The figure shows three views and two pictorial views of one solid part (mm, origin at its lowest corner). Answer the questions. Round coordinates to 2 decimals unless told otherwise and drop trailing zeros. Order: outer loops, then holes, each group sorted by start corner. A loop starts at its lowest first (then second) coordinate and runs counter-clockwise, first axis right, second up. Notation, with made-up numbers: (-14.5, 86.25) - (32.5, 86.25) arc R24 cw to (32.5, 104.25) - close; hole circle Ø6 at (75.5, 53). An arc over 180 degrees is marked (long way). One line per item, written item: value. Start each with the question number.
1. Section A-A, the plane x = 7.2 is taken. Give the vertices of the cut face in (y, z) (3 decimals).
2. Section C-C, the plane z = 1.75 is taken. Give the vertices of the cut face in (x, y) (3 decimals).
3. Section B-B, the plane y = 2.95 is taken. Give the vertices of the cut face in (x, z) (3 decimals).
4. Section D-D, the plane x = 56 is taken. Give the vertices of the cut face in (y, z), then the cut area to 3 significant figures.
5. Straight lines are drawn through the part: line 1 (Z direction, x = 50.5, y = 4.45); line 2 (X direction, y = 3.05, z = 1.5); line 3 (X direction, y = 4, z = 2.25). For each, find the intervals that lie inside material, in ascending order.
6. A flat-ended cylindrical pin translates along its axis: P1, Ø3, axis at x = 20.5, y = 2.5, coming from the -Z side. Find the tip coordinate at first contact, or state that the pin passes through.
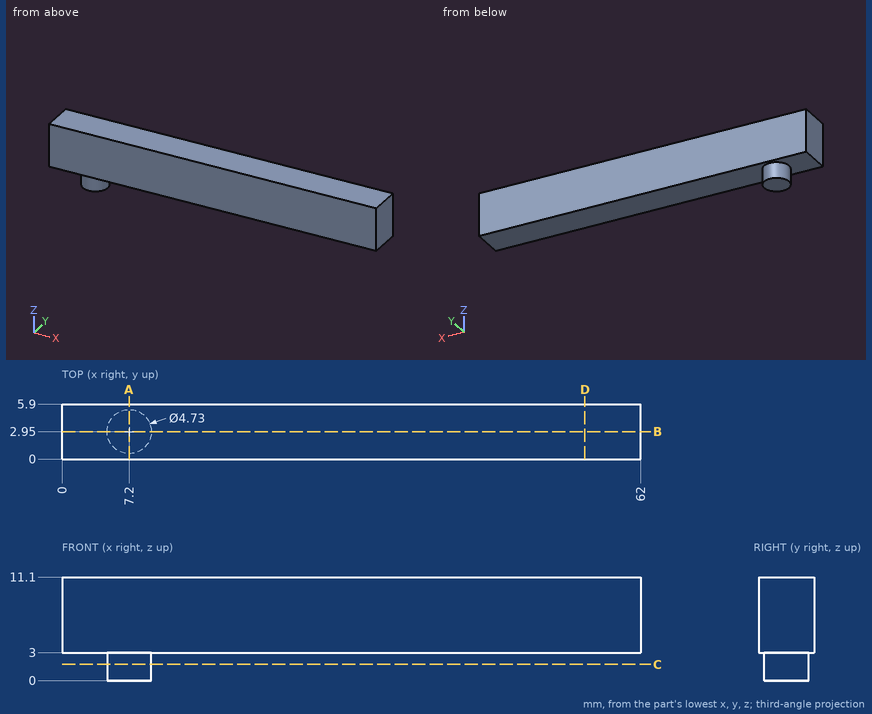
Answer list:
1. outline: (0, 3) - (0.585, 3) - (0.585, 0) - (5.315, 0) - (5.315, 3) - (5.9, 3) - (5.9, 11.1) - (0, 11.1) - close
2. outline: circle Ø4.73 at (7.2, 2.95)
3. outline: (0, 3) - (4.835, 3) - (4.835, 0) - (9.565, 0) - (9.565, 3) - (62, 3) - (62, 11.1) - (0, 11.1) - close
4. outline: (0, 3) - (5.9, 3) - (5.9, 11.1) - (0, 11.1) - close
4. area: 47.8 mm²
5. line 1: z = 3 to 11.1
5. line 2: x = 4.84 to 9.56
5. line 3: x = 5.08 to 9.32
6. P1: stops at z = 3
